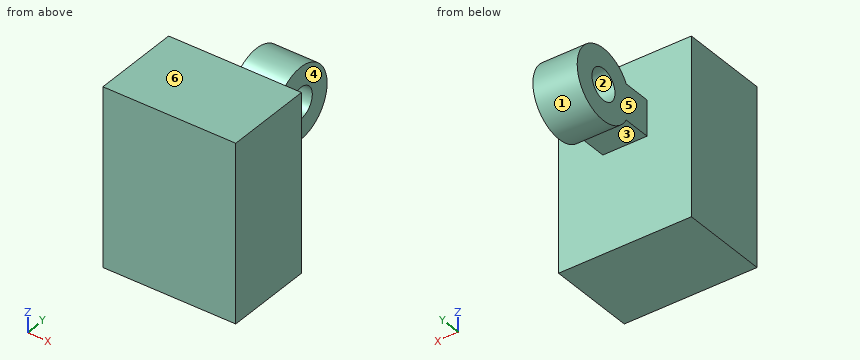
from build123d import *

# Parameters (mm, degrees)
ESQUISSE1_W        = 30
ESQUISSE1_H        = 20
BOSS_EXTRU_1_DEPTH = 40
ESQUISSE3_W        = 10
ESQUISSE3_H        = 8
BOSS_EXTRU_2_DEPTH = 8
ESQUISSE6_R        = 8
ESQUISSE6_R_2      = 3.5
BOSS_EXTRU_3_DEPTH = 10


with BuildPart() as part:
    # Esquisse1 → Boss.-Extru.1 (new body)
    with BuildSketch(Plane.XY):
        with Locations((-56.95643744, 10.673454793)):
            Rectangle(ESQUISSE1_W, ESQUISSE1_H)
    extrude(amount=BOSS_EXTRU_1_DEPTH)

    # Esquisse3 → Boss.-Extru.2 (add)
    with BuildSketch(Plane(origin=(0, 20.673454793, 0), x_dir=(1, 0, 0), z_dir=(0, 1, 0))):
        with Locations((-56.95643744, -26)):
            Rectangle(ESQUISSE3_W, ESQUISSE3_H)
    extrude(amount=BOSS_EXTRU_2_DEPTH)

    # Esquisse6 → Boss.-Extru.3 (add)
    with BuildSketch(Plane(origin=(-51.95643744, 0, 0), x_dir=(0, 0, -1), z_dir=(1, 0, 0))):
        with Locations((-26, 33.944580359)):
            Circle(ESQUISSE6_R)
        with Locations((-26, 33.944580359)):
            Circle(ESQUISSE6_R_2, mode=Mode.SUBTRACT)
    extrude(amount=-BOSS_EXTRU_3_DEPTH)


solid = part.part
Can you work these out from the model? Positions are in its coordinate system, mm. Face numbers are marked on the shaded views. A direction names the side the tool comes from. Give positions to 0.01 mm unless a question says otherwise; leave off trailing zeros. Write each loop counter-clockwise with the first axis right and the second up, starting at its lowest first coordinate (ties: lowest second). Pieces come first, ordered by that corner, then holes. Notation, with made-up numbers: M 50,54 L 84,54 A10 cw 84,68 Z; hole C 4.5,-16.75 d6. An arc over 180 degrees is marked long. Answer in a Markdown table with one row per item. Add a question column.
Item 1: Imagine slicing it at B-B, the plane x = -54.5. Write out the boundary of the cut face in (y, z), plus the area to 3 significant figures.
Item 2: Imagine slicing it at D-D, the plane y = 26. Write out the boundary of the cut face in (x, z).
Item 3: On a 3-axis mill with a long thin cutter (end or side, diameter ignored), from which of +Z, -Z, +X, -X, +Y, -Y can I reach the whole of each face in a straight line? I mean the marked faces 4, 5 and 6. Say none if no direction works.
Item 4: For pin 1 Ø2 at (x, z) = (-52, 14.5) entering from +Y; pin 2 Ø1.5 at (x, z) = (-57, 28) entering from +Y; pin 3 Ø1.9 at (x, y) = (-58, 24.5) entering from -Z, each with a flat end and sliding along its axis, tell me the tip position at first contact or that it passes through.
Item 5: We'd pull the mould along Z, two halves only. Please class the marked faces 1, 2 and 3: released by +Z, released by -Z, zero draft, split by the parting line, or undercut.
Item 6: Please list where these lines run through material, in increasing order: L1, parallel to Y at x = -67, z = 16; L2, parallel to Y at x = -56.25, z = 26; L3, parallel to X at y = 23.5, z = 24.
Item 7: Imagine slicing it at A-A, the plane z = 26. Write out the boundary of the cut face in (x, y), plus the area to 3 significant figures.
Item 8: Imagine slicing it at C-C, the plane z = 12.5. Write out the boundary of the cut face in (x, y).
Evaluation:
| question | item | result |
|---|---|---|
| 1 | outline | M 0.67,0 L 20.67,0 L 20.67,22 L 27.02,22 A8 ccw long 27.02,30 L 20.67,30 L 20.67,40 L 0.67,40 Z; hole C 33.94,26 d7 |
| 1 | area | 1,010 mm² |
| 2 | outline | M -61.96,22 L -51.96,22 L -51.96,30 L -61.96,30 Z |
| 3 | face 4 | +Z, -Z, +X, +Y |
| 3 | face 5 | +Z, -Z, -X, +Y |
| 3 | face 6 | +Z, +X, -X, +Y, -Y |
| 4 | pin 1 | stops at y = 20.67 |
| 4 | pin 2 | stops at y = 41.85 |
| 4 | pin 3 | stops at z = 22 |
| 5 | face 1 | split by the parting line |
| 5 | face 2 | undercut |
| 5 | face 3 | released by -Z |
| 6 | L1 | y = 0.67 to 20.67 |
| 6 | L2 | y = 0.67 to 30.44, 37.44 to 41.94 |
| 6 | L3 | x = -61.96 to -51.96 |
| 7 | outline | M -71.96,0.67 L -41.96,0.67 L -41.96,20.67 L -51.96,20.67 L -51.96,30.44 L -61.96,30.44 L -61.96,20.67 L -71.96,20.67 Z; M -61.96,37.44 L -51.96,37.44 L -51.96,41.94 L -61.96,41.94 Z |
| 7 | area | 743 mm² |
| 8 | outline | M -71.96,0.67 L -41.96,0.67 L -41.96,20.67 L -71.96,20.67 Z |
